Geometry check sheet. Reference: drawing and pictorial views, mm from the part's lowest x, y, z. Round coordinates to 2 decimals unless told otherwise and drop trailing zeros. Write each loop counter-clockwise with the first axis right and the second up, starting at its lowest first coordinate (ties: lowest second). Pieces come first, ordered by that corner, then holes. Notation, with made-up numbers: M -20.75,4 L 1.25,4 A30 ccw 1.25,42 Z; hole C -26.75,-14.5 d5. An arc over 180 degrees is marked long. Answer in a Markdown table with one row per item. Add a question column.
1. Go/stop test with flat-tipped pins: pin 1 Ø2.5 at (y, z) = (87, 3.5) entering from +X; pin 2 Ø2.5 at (x, z) = (88, 4.5) entering from +Y; pin 3 Ø2.5 at (x, y) = (3.5, 88) entering from +Z. Record where each tip stops, or that it passes through.
2. Material ranges on probe 1 along X at (y, z) = (87.5, 1.65), recorded low to high.
3. Sectioned sample at A-A on x = 87.5. Record the cut outline in (y, z), plus the area to 3 significant figures.
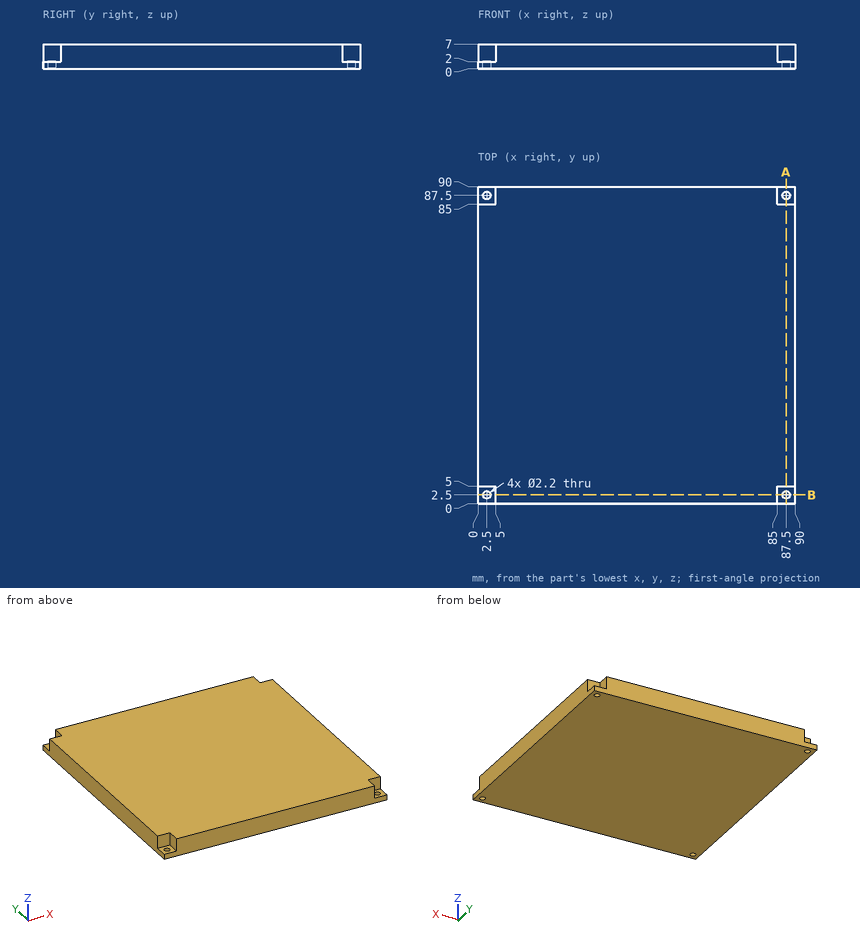
Geometry check:
| question | item | result |
|---|---|---|
| 1 | pin 1 | stops at x = 85 |
| 1 | pin 2 | stops at y = 85 |
| 1 | pin 3 | stops at z = 2 |
| 2 | probe 1 | x = 0 to 1.4, 3.6 to 86.4, 88.6 to 90 |
| 3 | outline | M 0,0 L 1.4,0 L 1.4,2 L 0,2 Z; M 3.6,0 L 86.4,0 L 86.4,2 L 85,2 L 85,7 L 5,7 L 5,2 L 3.6,2 Z; M 88.6,0 L 90,0 L 90,2 L 88.6,2 Z |
| 3 | area | 571 mm2 |
